Work out the finished part from the listing and answer in its coordinate system (mm). Face numbers are marked on the shaded views. A direction names the side the tool comes from. Coordinates: 2 decimals unless noted, no trailing zeros. Order: outer loops, then holes, each group sorted by start corner. A loop starts at its lowest first (then second) coordinate and runs counter-clockwise, first axis right, second up.
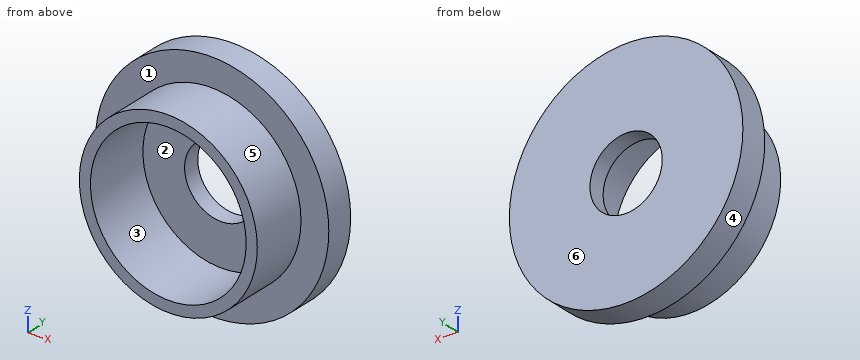
Autodesk Inventor part; units mm, degrees
ref_plane "YZ Plane" through (0, 0, 0) normal (1, 0, 0) x (0, 1, 0)
ref_plane "XZ Plane" through (0, 0, 0) normal (0, 1, 0) x (-1, 0, 0)
ref_plane "XY Plane" through (0, 0, 0) normal (0, 0, 1) x (1, 0, 0)
sketch "Sketch1" plane through (0, 0, 0) normal (0, 0, 1) x (1, 0, 0)
  line L0 (0, 0) -> (0, 13.3519) construction
  line L1 (14, -12) -> (14, 0)
  line L2 (14, 0) -> (6.5, 0)
  line L3 (6.5, 3) -> (21, 3)
  line L4 (21, 3) -> (21, -2)
  line L5 (21, -2) -> (16, -2)
  line L6 (16, -2) -> (16, -12)
  line L7 (16, -12) -> (14, -12)
  line L8 (6.5, 3) -> (6.5, 0)
  line L9 (0, 0) -> (6.5, 0) construction
  dimension "d0" = 28
  dimension "d1" = 12
  dimension "d2" = 10
  dimension "d3" = 32
  dimension "d4" = 5
  dimension "d5" = 42
  dimension "d9" = 13
revolve "Revolution1" add sketch "Sketch1" angle 360 about axis through (0, 0, 0) along (0, 1, 0)
thread "Thread1"
properties part number "LagerDeckel"
1. The part is cut by section A-A (z = 0). Determine the outline of the cut face in (x, y), plus the area to 3 significant figures.
2. The part is cut by section C-C (y = -1.25). Determine the outline of the cut face in (x, z), plus the area to 3 significant figures.
3. For the marked faces 5 and 6, determine the directions among +Z, -Z, +X, -X, +Y, -Y from which every point of the face is accessible in a straight line to the end or side of a thin tool.
4. The part is cut by section B-B (x = 0). Determine the outline of the cut face in (y, z), plus the area to 3 significant figures.
5. The part is cut by section D-D (x = -9.5). Determine the outline of the cut face in (y, z).
6. Flat-ended cylindrical pins translate along their axes: pin 1 (1.5 mm diameter, centred on y = -2, z = 6, fed in from -X); pin 2 (22.5 mm diameter, centred on x = 0, z = -4, fed in from -Y); pin 3 (5 mm diameter, centred on x = -13, y = -6.5, fed in from -Z); pin 4 (5 mm diameter, centred on y = -2, z = 10, fed in from -X). Find the tip coordinate at first contact, or state that the pin passes through.
7. Consider probe 1 along Z at (x, y) = (0, -5.25); probe 2 along X at (y, z) = (1, 0). Determine where each line is inside the solid, lowest interval first.
8. The mould has two halves that part along Z. Classify the marked faces 1, 2, 3 and 4: released by +Z, released by -Z, zero draft, split by the parting line, or undercut.
Worked out:
1. outline: (-21, -2) - (-16, -2) - (-16, -12) - (-14, -12) - (-14, 0) - (-6.5, 0) - (-6.5, 3) - (-21, 3) - close; (6.5, 0) - (14, 0) - (14, -12) - (16, -12) - (16, -2) - (21, -2) - (21, 3) - (6.5, 3) - close
1. area: 155 mm2
2. outline: circle Ø42 at (0, 0); hole circle Ø28 at (0, 0)
2. area: 770 mm2
3. face 5: -Y
3. face 6: +Z, -Z, +X, -X, +Y
4. outline: (-12, -16) - (-2, -16) - (-2, -21) - (3, -21) - (3, -6.5) - (0, -6.5) - (0, -14) - (-12, -14) - close; (-12, 14) - (0, 14) - (0, 6.5) - (3, 6.5) - (3, 21) - (-2, 21) - (-2, 16) - (-12, 16) - close
4. area: 155 mm2
5. outline: (-12, -12.87) - (-2, -12.87) - (-2, -18.73) - (3, -18.73) - (3, 18.73) - (-2, 18.73) - (-2, 12.87) - (-12, 12.87) - (-12, 10.28) - (0, 10.28) - (0, -10.28) - (-12, -10.28) - close
6. pin 1: stops at x = -20.33
6. pin 2: stops at y = -12
6. pin 3: stops at z = -12.07
6. pin 4: stops at x = -19.62
7. probe 1: z = -16 to -14, 14 to 16
7. probe 2: x = -21 to -6.5, 6.5 to 21
8. face 1: zero draft
8. face 2: undercut
8. face 3: undercut
8. face 4: split by the parting line
